```python
from build123d import *

# Parameters (mm, degrees)
SKETCH1_R           = 22
SKETCH1_R_2         = 19
BOSS_EXTRUDE1_DEPTH = 60
SKETCH2_R           = 22
BOSS_EXTRUDE2_DEPTH = 3
CUT_EXTRUDE1_DEPTH  = 40
SKETCH8_R           = 1.75
SKETCH8_W           = 3.317773355
SKETCH8_H           = 8.204416282
SKETCH8_W_2         = 3.240615835
SKETCH8_H_2         = 10.724895265
CUT_EXTRUDE4_DEPTH  = 68.586980995
SKETCH9_W           = 12
SKETCH9_H           = 4
BOSS_EXTRUDE3_DEPTH = 10
SKETCH10_R          = 1.75
CUT_EXTRUDE5_DEPTH  = 77.776729242


with BuildPart() as part:
    # Sketch1 → Boss-Extrude1 (new body)
    with BuildSketch(Plane.XY):
        Circle(SKETCH1_R)
        Circle(SKETCH1_R_2, mode=Mode.SUBTRACT)
    extrude(amount=BOSS_EXTRUDE1_DEPTH)

    # Sketch2 → Boss-Extrude2 (add)
    with BuildSketch(Plane.XY.offset(60)):
        Circle(SKETCH2_R)
    extrude(amount=BOSS_EXTRUDE2_DEPTH)

    # Sketch3 → Cut-Extrude1 (cut)
    with BuildSketch(Plane(origin=(0, 0, 0), x_dir=(-1, 0, 0), z_dir=(0, 0, -1))):
        with BuildLine():
            Line((-21.166010489, 6), (-18.027756377, 6))
            ThreePointArc((-18.027756377, 6), (-19, 0), (-18.027756377, -6))
            Line((-18.027756377, -6), (-21.166010489, -6))
            ThreePointArc((-21.166010489, -6), (-22, 0), (-21.166010489, 6))
        make_face()
        with BuildLine():
            Line((18.027756377, 6), (21.166010489, 6))
            ThreePointArc((21.166010489, 6), (22, 0), (21.166010489, -6))
            Line((21.166010489, -6), (18.027756377, -6))
            ThreePointArc((18.027756377, -6), (19, 0), (18.027756377, 6))
        make_face()
    extrude(amount=-CUT_EXTRUDE1_DEPTH, mode=Mode.SUBTRACT)

    # Sketch8 → Cut-Extrude4 (cut, through all)
    with BuildSketch(Plane(origin=(0, 0, 60), x_dir=(-1, 0, 0), z_dir=(0, 0, -1))):
        with Locations((-7.976328212, -7.816252109)):
            Circle(SKETCH8_R)
        with Locations((-7.976328212, 8.343747891)):
            Circle(SKETCH8_R)
        with Locations((8.253671788, 8.343747891)):
            Circle(SKETCH8_R)
        with Locations((8.253671788, -7.816252109)):
            Circle(SKETCH8_R)
        with Locations((6.962249116, -0.023129474)):
            Rectangle(SKETCH8_W, SKETCH8_H)
        with Locations((-6.681772319, -0.3831979)):
            Rectangle(SKETCH8_W_2, SKETCH8_H_2)
    extrude(amount=-CUT_EXTRUDE4_DEPTH, mode=Mode.SUBTRACT)

    # Sketch9 → Boss-Extrude3 (add)
    with BuildSketch(Plane(origin=(0, 0, 0), x_dir=(-1, 0, 0), z_dir=(0, 0, -1))):
        with Locations((-24.027756377, 8)):
            Rectangle(SKETCH9_W, SKETCH9_H)
        with Locations((-24.027756377, -8)):
            Rectangle(SKETCH9_W, SKETCH9_H)
        with Locations((24.027756377, -8)):
            Rectangle(SKETCH9_W, SKETCH9_H)
        with Locations((24.027756377, 8)):
            Rectangle(SKETCH9_W, SKETCH9_H)
    extrude(amount=-BOSS_EXTRUDE3_DEPTH)

    # Sketch10 → Cut-Extrude5 (cut, through all)
    with BuildSketch(Plane(origin=(0, 10, 0), x_dir=(1, 0, 0), z_dir=(0, 1, 0))):
        with Locations(Location((-26.027756377, -5, 0), (0, 0, 180))):
            Circle(SKETCH10_R)
        with Locations((26.027756377, -5)):
            Circle(SKETCH10_R)
    extrude(amount=-CUT_EXTRUDE5_DEPTH, mode=Mode.SUBTRACT)


solid = part.part
```
Model file for the job. Use its own axes, mm. A direction names the side the tool comes from. Give positions to 0.01 mm unless a question says otherwise; leave off trailing zeros. Loops run counter-clockwise (first coordinate to the right, second up) from the corner with the lowest first, then second, coordinate; pieces in that order, holes last. Notation, with made-up numbers: (69.25, 5) - (109.25, 5) arc R12 cw to (109.25, 10) - close; hole circle Ø6 at (54, 7). An arc over 180 degrees is marked (long way). One line per item, written item: value. Start each with the question number.
1. Probe L1, parallel to Y at x = 26.5, z = 8; L2, parallel to X at y = 6.5, z = 4; L3, parallel to Z at x = 12, y = -2.5. List the from-to ranges inside material, lowest first. Write a range as from..to.
2. Pull direction Z, two halves, no side cores. Call faces 1 (the flat face through (25, 8, 10)), 2 (the cylindrical face through (27.644, 8.028, 5.67)), 3 (the flat face through (7, 4.979, 61)): pulls with the +Z half, pulls with the -Z half, needs draft (parallel to the pull), parting line crosses it, or undercut.
3. Slice it at B-B (y = 0). List the corners of the cut face in (x, z), plus the area to 3 significant figures.
4. Slice it at D-D (y = -15). List the corners of the cut face in (x, z), plus the area to 3 significant figures.
5. Which spindle directions (+Z, -Z, +X, -X, +Y, -Y) get a long thin tool onto all of the face, cutting with end or side? Do faces 4 (the cylindrical face through (20.984, 6.608, 31.059)), 5 (the flat face through (5.061, 0, 61)), 6 (the flat face through (0, 0, 60)), 7 (the flat face through (-20, 6, 15)). Say none if no direction does.
6. Slice it at A-A (z = 5). Give the number of separate pieces and of enclosed holes in the cut face, plus the area to 3 significant figures.
7. Pin check, flat tips, straight feed: pin 1 (3 mm diameter, centred on y = -7, z = 23, fed in from +X); pin 2 (12 mm diameter, centred on y = 15.5, z = 35.5, fed in from +X); pin 3 (9.5 mm diameter, centred on x = -22, z = 23, fed in from -Y). Stop position of each tip, or through.
8. Slice it at C-C (x = -11). List the corners of the cut face in (y, z).
Solution:
1. L1: y = -10..-6, 6..10
1. L2: x = -30.03..-27.46, -24.59..-17.85, 17.85..24.59, 27.46..30.03
1. L3: z = 60..63
2. face 1: pulls with the +Z half
2. face 2: undercut
2. face 3: needs draft
3. outline: (-22, 40) - (-19, 40) - (-19, 60) - (-8.62, 60) - (-8.62, 63) - (-22, 63) - close; (-5.3, 60) - (5.06, 60) - (5.06, 63) - (-5.3, 63) - close; (8.3, 60) - (19, 60) - (19, 40) - (22, 40) - (22, 63) - (8.3, 63) - close
3. area: 232 mm^2
4. outline: (-16.09, 0) - (-11.66, 0) - (-11.66, 60) - (11.66, 60) - (11.66, 0) - (16.09, 0) - (16.09, 63) - (-16.09, 63) - close
4. area: 628 mm^2
5. face 4: +Z
5. face 5: +Z, -Z
5. face 6: -Z
5. face 7: -Z, +X, -X
6. separate pieces: 6
6. enclosed holes: 0
6. area: 410 mm^2
7. pin 1: stops at x = 21.17
7. pin 2: stops at x = 19.84
7. pin 3: stops at y = -13.65
8. outline: (-19.05, 0) - (-15.49, 0) - (-15.49, 60) - (15.49, 60) - (15.49, 0) - (19.05, 0) - (19.05, 63) - (-19.05, 63) - close
